For this review, take the finished solid that the model builds, in its own axes (mm). A direction names the side the tool comes from. Coordinates: 2 decimals unless noted, no trailing zeros. Loops run counter-clockwise (first coordinate to the right, second up) from the corner with the lowest first, then second, coordinate; pieces in that order, holes last. Notation, with made-up numbers: M 38.25,66 L 91.25,66 A26 ccw 91.25,94 Z; hole C 37,49.25 d4. An arc over 180 degrees is marked long. Answer as a JSON object with one key per item and string values. Group by question number.
Item 1: Insertion check: pin 1 (1 mm diameter, centred on y = 35, z = -5, fed in from +X); pin 2 (4 mm diameter, centred on y = 33.5, z = -2.5, fed in from -X); pin 3 (2 mm diameter, centred on x = -3.5, y = 39, fed in from -Z). Each pin has a flat end and moves straight along its axis. Give the tip position at first contact, or say it passes through.
Item 2: Add section C-C (z = -3). State the section outline as (x, y) points, then the cut area to 3 significant figures.
Item 3: Mouldability with a two-part tool opening along X and no side actions: class faces 6 (the face through (-4, 37, -1)), 7 (the face through (-4.12, 44.99, -3.54)), 8 (the face through (0, 13, -9)) as +X half, -X half, draft (parallel to the pull), parting line (faces both ways), or undercut.
Item 4: Tool access review of faces 1 (the face through (-4, 37, -6)), 2 (the face through (-7.75, 37, -4)), 3 (the face through (-0.75, 37, -3)), 4 (the face through (-4, 13, -17)), 5 (the face through (-4, 0, -8)): name each direction out of +Z, -Z, +X, -X, +Y, -Y from which nothing blocks a thin tool from reaching the whole face with its end or side.
Item 5: Add section D-D (x = -6.5). State the section outline as (y, z) points, then the cut area to 3 significant figures.
Item 6: Add section B-B (x = -4.25). State the section outline as (y, z) points, then the cut area to 3 significant figures.
Item 7: Add section A-A (y = 44). State the section outline as (x, z) points.
Item 8: Wall thickness on L1, parallel to Y at x = -4.25, z = -3.5; L2, parallel to Y at x = -3, z = -15.25; L3, parallel to Z at x = -1.5, y = 41: over which ranges is each line inside the solid? List them lowest first. Write a range as from..to.
Autodesk Inventor part; units mm, degrees
ref_plane "YZ Plane" through (0, 0, 0) normal (1, 0, 0) x (0, 1, 0)
ref_plane "XZ Plane" through (0, 0, 0) normal (0, 1, 0) x (-1, 0, 0)
ref_plane "XY Plane" through (0, 0, 0) normal (0, 0, 1) x (1, 0, 0)
sketch "Sketch1" plane through (0, 0, 0) normal (0, 1, 0) x (-1, 0, 0)
  line L0 (0, 0) -> (8.5, 0)
  line L1 (8.5, 0) -> (8.5, -17)
  line L2 (8.5, -17) -> (0, -17)
  line L3 (0, -17) -> (0, 0)
  dimension "d0" = 8.5
  dimension "d1" = 17
extrude "Extrusion1" add sketch "Sketch1" along normal blind 27
sketch "Sketch2" plane through (0, 27, 0) normal (0, 1, 0) x (1, 0, 0)
  line L0 (-7.75, 1) -> (-0.75, 1)
  line L1 (-0.75, 1) -> (-0.75, 6)
  line L2 (-0.75, 6) -> (-7.75, 6)
  line L3 (-7.75, 6) -> (-7.75, 1)
  line L4 (-8.5, 0) -> (0, 0)
  line L5 (-8.5, 17) -> (-8.5, 0)
  dimension "d4" = 7
  dimension "d5" = 5
  dimension "d6" = 1
  dimension "d7" = 0.75
extrude "Extrusion2" add sketch "Sketch2" along normal blind 20
sketch "Sketch3" plane through (-0.75, 27, -6) normal (0, 0, -1) x (-1, 0, 0)
  circle A0 centre (3.5, 17) radius 1
  line L0 (7, 0) -> (7, 20)
  line L1 (-0.75, 0) -> (7.75, 0)
  point P0 (-0.75, -27)
  dimension "d10" = 2
  dimension "d11" = 3.5
  dimension "d12" = 17
extrude "Extrusion3" cut sketch "Sketch3" against normal through all
properties part number "support_axe_radio"
From the geometry:
{
 "1": {"pin 1": "stops at x = -0.75", "pin 2": "stops at x = -7.75", "pin 3": "stops at z = -6"},
 "2": {"outline": "M -8.5,0 L 0,0 L 0,27 L -0.75,27 L -0.75,47 L -7.75,47 L -7.75,27 L -8.5,27 Z; hole C -4.25,44 d2", "area": "366 mm²"},
 "3": {"face 6": "draft", "face 7": "undercut", "face 8": "+X half"},
 "4": {"face 1": "-Z, +X, -X, +Y", "face 2": "+Z, -Z, -X, +Y", "face 3": "+Z, -Z, +X, +Y", "face 4": "-Z, +X, -X, +Y, -Y", "face 5": "+Z, -Z, +X, -X, -Y"},
 "5": {"outline": "M 0,-17 L 27,-17 L 27,-6 L 47,-6 L 47,-1 L 27,-1 L 27,0 L 0,0 Z", "area": "559 mm²"},
 "6": {"outline": "M 0,-17 L 27,-17 L 27,-6 L 43,-6 L 43,-1 L 27,-1 L 27,0 L 0,0 Z; M 45,-6 L 47,-6 L 47,-1 L 45,-1 Z", "area": "549 mm²"},
 "7": {"outline": "M -7.75,-6 L -5.25,-6 L -5.25,-1 L -7.75,-1 Z; M -3.25,-6 L -0.75,-6 L -0.75,-1 L -3.25,-1 Z"},
 "8": {"L1": "y = 0..43, 45..47", "L2": "y = 0..27", "L3": "z = -6..-1"}
}
